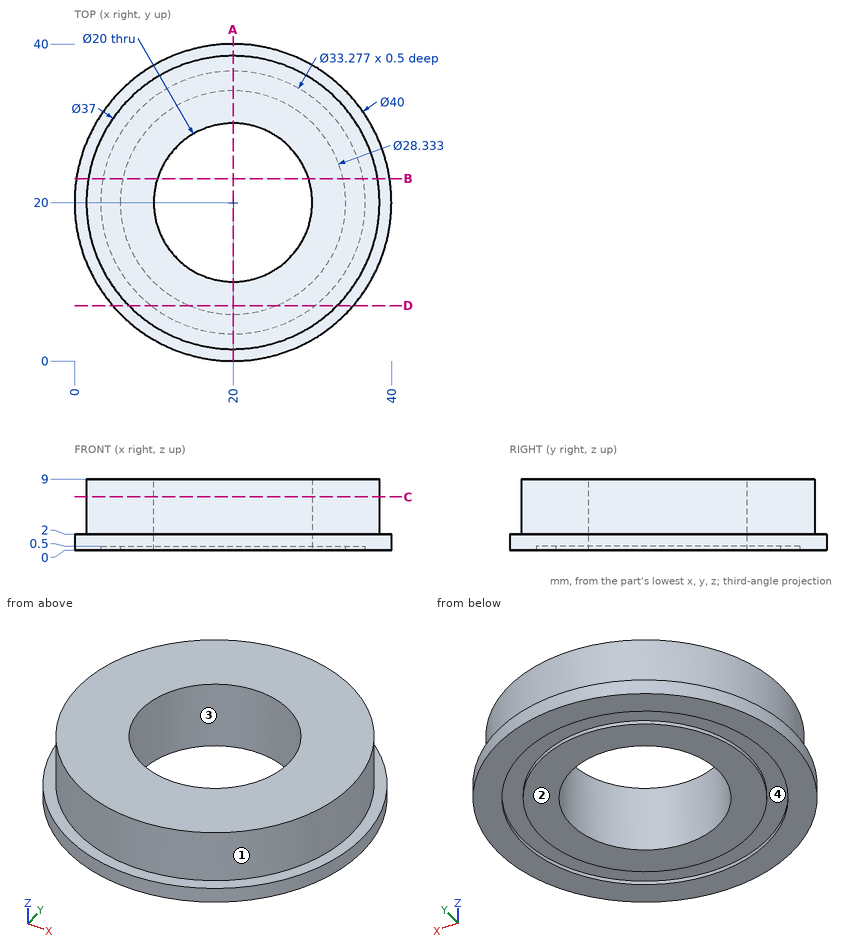
Source: three-view drawing plus pictorial views. Frame: mm from the lowest corner of the part. Round coordinates to 2 decimals unless told otherwise and drop trailing zeros. Loops run counter-clockwise (first coordinate to the right, second up) from the corner with the lowest first, then second, coordinate; pieces in that order, holes last. Notation, with made-up numbers: M 30,11.25 L 40,11.25 A24 cw 40,45.25 Z; hole C -18,26.5 d11. An arc over 180 degrees is marked long. Put each result on its own line as item: value.
(1) First-contact query: pin 1 (3 mm diameter, centred on y = 32, z = 5, fed in from -X); pin 2 (12 mm diameter, centred on x = 27.5, y = 10, fed in from -Z); pin 3 (2 mm diameter, centred on x = 19, z = 1, fed in from -Y); pin 4 (4 mm diameter, centred on y = 12.5, z = 4.5, fed in from -X). Flat tips, straight axial feed; report the tip coordinate or a pass-through.
Solutions:
pin 1: x = 4.77
pin 2: z = 0
pin 3: y = 0
pin 4: x = 2.34
(2) Section D-D, the plane y = 7. Return loops of the section in (x, z) (1 decimal).
Solutions:
outline: M 4.8,0 L 9.6,0 L 9.6,0.5 L 14.4,0.5 L 14.4,0 L 25.6,0 L 25.6,0.5 L 30.4,0.5 L 30.4,0 L 35.2,0 L 35.2,2 L 33.2,2 L 33.2,9 L 6.8,9 L 6.8,2 L 4.8,2 Z
(3) Section B-B, the plane y = 23. Return loops of the section in (x, z) (1 decimal).
Solutions:
outline: M 0.2,0 L 3.6,0 L 3.6,0.5 L 6.2,0.5 L 6.2,0 L 10.5,0 L 10.5,9 L 1.7,9 L 1.7,2 L 0.2,2 Z; M 29.5,0 L 33.8,0 L 33.8,0.5 L 36.4,0.5 L 36.4,0 L 39.8,0 L 39.8,2 L 38.3,2 L 38.3,9 L 29.5,9 Z
(4) Section A-A, the plane x = 20. Return loops of the section in (y, z).
Solutions:
outline: M 0,0 L 3.36,0 L 3.36,0.5 L 5.83,0.5 L 5.83,0 L 10,0 L 10,9 L 1.5,9 L 1.5,2 L 0,2 Z; M 30,0 L 34.17,0 L 34.17,0.5 L 36.64,0.5 L 36.64,0 L 40,0 L 40,2 L 38.5,2 L 38.5,9 L 30,9 Z
(5) Section C-C, the plane z = 6.75. Return loops of the section in (x, y).
Solutions:
outline: C 20,20 d37; hole C 20,20 d20
(6) Pull-direction query (Y, two-part tool) for the marked faces 1, 2, 3 and 4; classes: released by +Y, released by -Y, zero draft, split by the parting line, or undercut.
Solutions:
face 1: split by the parting line
face 2: zero draft
face 3: undercut
face 4: undercut
(7) Ray query, line 1 (Y direction, x = 20, z = 0.2); line 2 (Y direction, x = 20, z = 6.75); line 3 (X direction, y = 28, z = 4.5). Return the intervals inside material, ascending. Write a range as [from, to].
Solutions:
line 1: [0, 3.36], [5.83, 10], [30, 34.17], [36.64, 40]
line 2: [1.5, 10], [30, 38.5]
line 3: [3.32, 14], [26, 36.68]
